Autodesk Inventor part; units mm, degrees
ref_plane "Work Plane2" through (3.35, 0, 0) normal (0, 0, -1) x (1, 0, 0)
ref_plane "YZ Plane" through (0, 0, 0) normal (1, 0, 0) x (0, 1, 0)
ref_plane "XZ Plane" through (0, 0, 0) normal (0, 1, 0) x (-1, 0, 0)
sketch "Sketch1" plane through (0, 0, 0) normal (0, 0, 1) x (1, 0, 0)
  line L0 (2.1, 0) -> (10, 0)
  line L1 (10, 0) -> (10, 1.5)
  line L2 (10, 1.5) -> (2.65, 1.5)
  line L3 (2.65, 1.5) -> (2.3433, 1.3466)
  line L4 (2.3433, 1.3466) -> (1.9814, 1.3466)
  line L5 (0, 2.75) -> (0, 1.6)
  line L6 (0, 1.6) -> (1.6999, 0.7525)
  line L7 (1.6999, 0.7525) -> (2.1, 0)
  line L8 (-2, 0) -> (12, 0)
  line L9 (0, -0.55) -> (0, 3.3)
  line L10 (0, 2.75) -> (0.2466, 2.75)
  line L11 (0.2466, 2.75) -> (1.4157, 1.581)
  line L12 (2.65, 1.5) -> (1.4966, 1.5) construction
  arc A0 (1.4157, 1.581) -> (1.9814, 1.3466) centre (1.9814, 2.1466) ccw
  point P0 (1.65, 1.3466)
  dimension "d1" = 7.35
  dimension "d2" = 3
  dimension "d3" = 2.6933
  dimension "d4" = 3.2
  dimension "d5" = 26.5
  dimension "d6" = 62
  dimension "d7" = 2.1
  dimension "d8" = 0.3067
  dimension "d12" = 5.5
  dimension "d13" = 45
  dimension "d15" = 10
  dimension "d24" = 1.65
  dimension "d93" = 0.8
revolve "Body" add sketch "Sketch1" angle 360 about axis through (2.1, 0, 0) along (1, 0, 0) contours L7 L6 L5 L10 L11 A0 L4 L3 L2 L1 L0
sketch "Sketch2" plane through (0, 0, 0) normal (-1, 0, 0) x (0, 0, 1)
  line L0 (0, 1.6) -> (0, 0) construction
  line L1 (0, 0) -> (1.6, 0) construction
  arc A0 (0.48, 0) -> (0, 0.48) centre (0, 0) ccw construction
  arc A1 (0.56, 0) -> (0, 0.56) centre (0, 0) ccw construction
  arc A2 (1.5795, 0.255) -> (0.255, 1.5795) centre (0, 0) ccw
  line L2 (0, 0) -> (1.1314, 1.1314) construction
  line L3 (0.255, 1.5795) -> (0.2766, 0.4869)
  line L4 (1.5795, 0.255) -> (0.4869, 0.2766)
  arc A3 (0.255, 1.5795) -> (0, 1.6) centre (0, 0) ccw
  arc A4 (1.6, 0) -> (1.5795, 0.255) centre (0, 0) ccw
  line L5 (0, -3.85) -> (0, 3.85)
  line L6 (-3.85, 0) -> (3.85, 0)
  arc A5 (0.255, -1.5795) -> (1.5795, -0.255) centre (0, 0) ccw
  line L7 (0.255, -1.5795) -> (0.2766, -0.4869)
  line L8 (1.5795, -0.255) -> (0.4869, -0.2766)
  arc A6 (0, -1.6) -> (0.255, -1.5795) centre (0, 0) ccw
  arc A7 (1.5795, -0.255) -> (1.6, 0) centre (0, 0) ccw
  arc A8 (-0.255, 1.5795) -> (-1.5795, 0.255) centre (0, 0) ccw
  line L9 (-0.255, 1.5795) -> (-0.2766, 0.4869)
  line L10 (-1.5795, 0.255) -> (-0.4869, 0.2766)
  arc A9 (0, 1.6) -> (-0.255, 1.5795) centre (0, 0) ccw
  arc A10 (-1.5795, 0.255) -> (-1.6, 0) centre (0, 0) ccw
  arc A11 (-0.255, -1.5795) -> (0, -1.6) centre (0, 0) ccw
  arc A12 (-1.5795, -0.255) -> (-0.255, -1.5795) centre (0, 0) ccw
  arc A13 (-1.6, 0) -> (-1.5795, -0.255) centre (0, 0) ccw
  line L11 (-1.5795, -0.255) -> (-0.4869, -0.2766)
  line L12 (-0.255, -1.5795) -> (-0.2766, -0.4869)
  arc A14 (0.2766, 0.4869) -> (0.4869, 0.2766) centre (0.4912, 0.4912) ccw
  arc A15 (0.4869, -0.2766) -> (0.2766, -0.4869) centre (0.4912, -0.4912) ccw
  arc A16 (-0.4869, 0.2766) -> (-0.2766, 0.4869) centre (-0.4912, 0.4912) ccw
  arc A17 (-0.2766, -0.4869) -> (-0.4869, -0.2766) centre (-0.4912, -0.4912) ccw
  point P0 (1.1314, -1.1314)
  point P1 (-1.1314, 1.1314)
  point P2 (-1.1314, -1.1314)
  dimension "d17" = 0.96
  dimension "d18" = 1.12
  dimension "d19" = 3.2
  dimension "d20" = 45
  dimension "d21" = 0.255
extrude "Slot" add sketch "Sketch2" against normal up to next draft 5 contours L4 A14 L3 A2 | A5 L7 A15 L8 | L9 A16 L10 A8 | A12 L11 A17 L12
fillet "Fillet1" radius 0.102 4 edges at (0, 1.6, 0) (0, 0, -1.6) (0, -1.6, 0) (0, 0, 1.6)
thread "Thread"
chamfer "Chamfer1" distance 0.3067 distance2 0.3069 1 edges at (10, -1.5, 0) measured on face at (10, -0.5112, 0.3316)
ref_plane "Work Plane2" through (3.35, 0, 0) normal (0, 0, -1) x (1, 0, 0)
equation "\"d17\" = 0.3 * SDM"
equation "\"d18\" = 0.35 * SDM"
equation "\"d19\" = SDM"
equation "\"d21\" = 0.5 * SBR"
equation "\"d1\" = GEL"
equation "\"d2\" = GD"
equation "\"d3\" = BDM"
equation "\"d4\" = SDM"
equation "\"d7\" = INTI"
equation "\"d8\" = GAL"
equation "\"d12\" = KOD"
equation "\"d13\" = 0.5 * SEWI"
equation "\"d15\" = NLG"
equation "\"d93\" = R"
equation "\"d23\" = 0.2 * SBR"
equation "\"d10\" = GEL"
equation "\"d25\" = -0.5 * SPD + 0.5 * GD"
equation "\"NLG\" = 10"
equation "\"GEL\" = 7.35"
equation "\"GAL\" = 0.61345 * PTC"
equation "\"SPD\" = NND - 1.2269 * PTC"
equation "\"KOD\" = 5.5"
equation "\"KOH\" = 1.65"
equation "\"SBR\" = 0.51"
equation "\"INTI\" = 2.1"
equation "\"SDM\" = 3.2"
equation "\"GD\" = NND"
equation "\"BDM\" = NND - GAL"
equation "\"SEWI\" = 90deg"
equation "\"d9\" = SDM"
equation "\"R\" = 0.8"
equation "\"GUL\" = 0.61345 * PTC"
equation "\"TOA\" = 30deg"
equation "\"EPV\" = 3.15"
equation "\"THREADDIA\" = 3"
equation "\"PTC\" = 0.5"
equation "\"NND\" = 3"
equation "\"GD1\" = THREADDIA - 1.2269 * PTC"
properties part number "ISO 7046-1  - M3 x 10 - 4.8 - H" material "Steel"
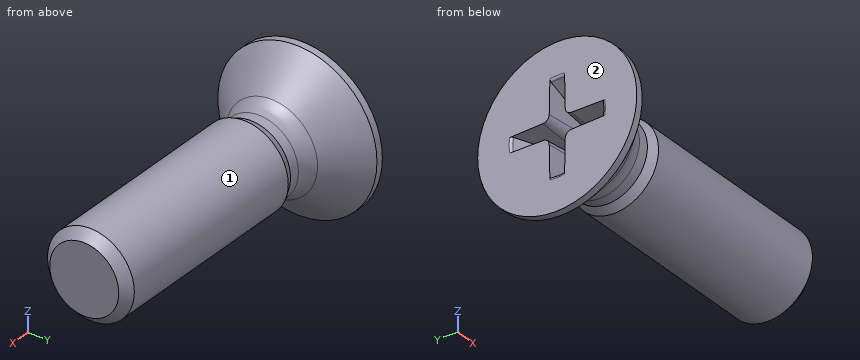
The listing builds one solid part. Answer for the finished solid, in the listing's coordinates (mm). Face numbers are marked on the shaded views. A direction names the side the tool comes from. Give positions to 0.01 mm unless a question says otherwise; leave off trailing zeros. Order: outer loops, then holes, each group sorted by start corner. A loop starts at its lowest first (then second) coordinate and runs counter-clockwise, first axis right, second up.
Item 1: Find the intervals of material crossed by probe 1 along Y at (x, z) = (4, 0.1); probe 2 along X at (y, z) = (2.15, 0.65); probe 3 along Z at (x, y) = (0.5, -1), in increasing order.
From the geometry:
probe 1: y = -1.5 to 1.5
probe 2: x = 0 to 0.75
probe 3: z = -2.29 to -0.22, 0.22 to 2.29
Item 2: The part is cut by section A-A, the plane x = 3.5. Give the vertices of the cut face in (y, z), and give its area (3 significant figures).
From the geometry:
outline: circle Ø3 at (0, 0)
area: 7.07 mm2
Item 3: Given pin 1 Ø1.5 at (x, z) = (2.5, -1) entering from +Y; pin 2 Ø2 at (x, z) = (1.5, -0.5) entering from +Y, each flat-ended and moving along its own axis, determine where each tip first touches the part or whether it passes through.
From the geometry:
pin 1: stops at y = 1.48
pin 2: stops at y = 2.46
Item 4: Which of the six approach directions +Z, -Z, +X, -X, +Y, -Y give full straight-line access (tool end or side, diameter ignored) to the marked faces 1 and 2?
From the geometry:
face 1: +X
face 2: +Z, -Z, -X, +Y, -Y
